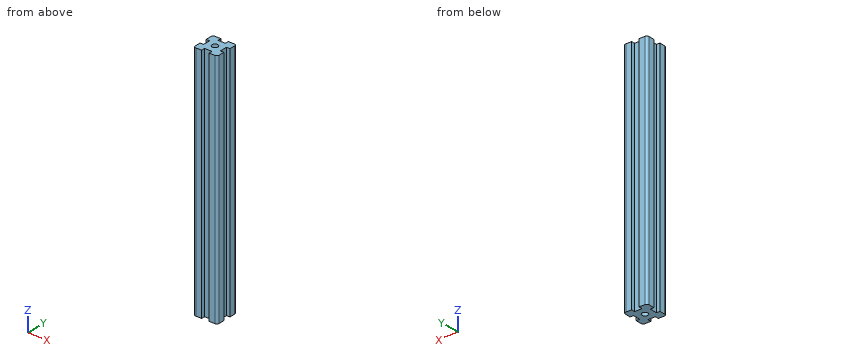
Autodesk Inventor part; units mm, degrees
ref_plane "YZ Plane" through (0, 0, 0) normal (1, 0, 0) x (0, 1, 0)
ref_plane "XZ Plane" through (0, 0, 0) normal (0, 1, 0) x (-1, 0, 0)
ref_plane "XY Plane" through (0, 0, 0) normal (0, 0, 1) x (1, 0, 0)
sketch "Sketch1" plane through (0, 0, 0) normal (0, 0, 1) x (1, 0, 0)
  line L0 (-10, 10) -> (-3.15, 10)
  line L1 (-3.15, 10) -> (-3.15, 7)
  line L2 (-3.15, 7) -> (3.15, 7)
  line L3 (3.15, 7) -> (3.15, 10)
  line L4 (3.15, 10) -> (10, 10)
  line L5 (10, 10) -> (10, 3.15)
  line L6 (10, 3.15) -> (7, 3.15)
  line L7 (7, 3.15) -> (7, -3.15)
  line L8 (7, -3.15) -> (10, -3.15)
  line L9 (10, -3.15) -> (10, -10)
  line L10 (10, -10) -> (3.15, -10)
  line L11 (3.15, -10) -> (3.15, -7)
  line L12 (3.15, -7) -> (-3.15, -7)
  line L13 (-3.15, -7) -> (-3.15, -10)
  line L14 (-10, -10) -> (-10, -3.15)
  line L15 (-10, -3.15) -> (-7, -3.15)
  line L16 (-7, -3.15) -> (-7, 3.15)
  line L17 (-7, 3.15) -> (-10, 3.15)
  line L18 (-10, 10) -> (-10, 3.15)
  line L19 (-3.15, -10) -> (-10, -10)
  circle A0 centre (0, 0) radius 2.5
  point P0 (0, 7)
  point P1 (-7, 0)
  dimension "d0" = 20
  dimension "d1" = 6.3
  dimension "d2" = 3
  dimension "d3" = 5
extrude "Extrusion1" add sketch "Sketch1" along normal mid plane 200
fillet "Fillet1" radius 2 4 edges at (-10, 10, 0) (10, 10, 0) (10, -10, 0) (-10, -10, 0)
properties part number "Profil"
Build history of the part. All positions in model axes, mm. Round coordinates to 2 decimals unless told otherwise and drop trailing zeros. Write each loop counter-clockwise with the first axis right and the second up, starting at its lowest first coordinate (ties: lowest second). Pieces come first, ordered by that corner, then holes. Notation, with made-up numbers: (37.5, 16) - (66.5, 16) arc R21 cw to (66.5, 31) - close; hole circle Ø2 at (87.5, -19.5). An arc over 180 degrees is marked (long way). Use CSV: the item, a comma, the result in double quotes.
(1) Band-saw the part on A-A (y = 0). Write the cut outline in (x, z).
Response:
outline,"(-7, -100) - (-2.5, -100) - (-2.5, 100) - (-7, 100) - close; (2.5, -100) - (7, -100) - (7, 100) - (2.5, 100) - close"
(2) Wall check: line 1 (Y direction, x = 0, z = -34); line 2 (X direction, y = 7.25, z = -19). Give the ranges that are in metal, low to high.
Response:
line 1,"-7 to -2.5, 2.5 to 7"
line 2,"-10 to -3.15, 3.15 to 10"
(3) Band-saw the part on B-B (z = -39). Write the cut outline in (x, y).
Response:
outline,"(-10, -8) arc R2 ccw to (-8, -10) - (-3.15, -10) - (-3.15, -7) - (3.15, -7) - (3.15, -10) - (8, -10) arc R2 ccw to (10, -8) - (10, -3.15) - (7, -3.15) - (7, 3.15) - (10, 3.15) - (10, 8) arc R2 ccw to (8, 10) - (3.15, 10) - (3.15, 7) - (-3.15, 7) - (-3.15, 10) - (-8, 10) arc R2 ccw to (-10, 8) - (-10, 3.15) - (-7, 3.15) - (-7, -3.15) - (-10, -3.15) - close; hole circle Ø5 at (0, 0)"
(4) Pin check, flat tips, straight feed: P1, Ø3, axis at y = 1.5, z = -31.5, coming from the -X side; P2, Ø3, axis at x = -1, z = -2.5, coming from the -Y side. Stop position of each tip, or through.
Response:
P1,"x = -7"
P2,"y = -7"
